Geometry: final body of the model. Coordinates: model frame, mm. A direction names the side the tool comes from. Give positions to 0.01 mm unless a question says otherwise; leave off trailing zeros. Loops run counter-clockwise (first coordinate to the right, second up) from the corner with the lowest first, then second, coordinate; pieces in that order, holes last. Notation, with made-up numbers: (5, -15) - (10, -15) arc R16 cw to (10, 3) - close; hole circle Ø1 at (-8.75, -11). An arc over 180 degrees is marked (long way). Answer in a Markdown table with one row per item.
from build123d import *
from OCP.BRepFilletAPI import BRepFilletAPI_MakeChamfer

# Parameters (mm, degrees)
SKETCH1_W            = 85
SKETCH1_H            = 23.9
BOSS_EXTRUDE1_DEPTH  = 1.7
SKETCH2_R            = 1.025
CUT_EXTRUDE1_DEPTH   = 45.180793338
SKETCH3_W            = 12
SKETCH3_H            = 6
BOSS_EXTRUDE2_DEPTH  = 5.6
SKETCH4_W            = 0.7
SKETCH4_H            = 1.5
BOSS_EXTRUDE3_DEPTH  = 3.6
CHAMFER1_SIZE        = 1.5
CHAMFER1_SIZE_2      = 1
SKETCH5_W            = 12
SKETCH5_H            = 5.6
CUT_EXTRUDE2_DEPTH   = 0.1
SKETCH6_W            = 10.2
SKETCH6_H            = 4.6
BOSS_EXTRUDE4_DEPTH  = 2.8
SKETCH7_R            = 0.7
BOSS_EXTRUDE5_DEPTH  = 5.8
BOSS_EXTRUDE6_DEPTH  = 3.65
SKETCH9_R            = 6.925
BOSS_EXTRUDE7_DEPTH  = 4.9
SKETCH10_R           = 5.95
BOSS_EXTRUDE8_DEPTH  = 4
SKETCH11_R           = 7
BOSS_EXTRUDE9_DEPTH  = 2.65
SKETCH12_R           = 4.5
CUT_EXTRUDE3_DEPTH   = 1
SKETCH13_R           = 4.45
BOSS_EXTRUDE10_DEPTH = 1.5
FILLET1_R            = 4.45
SKETCH14_W           = 13.1
SKETCH14_H           = 4.5
BOSS_EXTRUDE11_DEPTH = 2
SKETCH15_W           = 8
SKETCH15_H           = 0.5
BOSS_EXTRUDE12_DEPTH = 3


# Some blends are built 0.0001 mm under size
with BuildPart() as part:
    # Sketch1 → Boss-Extrude1 (new body)
    with BuildSketch(Plane(origin=(0, 0, 0), x_dir=(1, 0, 0), z_dir=(0, 1, 0))):
        Rectangle(SKETCH1_W, SKETCH1_H)
    extrude(amount=BOSS_EXTRUDE1_DEPTH)

    # Sketch2 → Cut-Extrude1 (cut, through all)
    with BuildSketch(Plane(origin=(0, 1.7, 0), x_dir=(1, 0, 0), z_dir=(0, 1, 0))):
        with Locations(Location((-40.605, 3.345, 0), (0, 0, 270))):
            Circle(SKETCH2_R)
        with Locations(Location((-10.45, 3.345, 0), (0, 0, 270))):
            Circle(SKETCH2_R)
        with Locations(Location((-40.605, -10.055, 0), (0, 0, 270))):
            Circle(SKETCH2_R)
        with Locations(Location((-10.45, -10.055, 0), (0, 0, 270))):
            Circle(SKETCH2_R)
        with Locations(Location((10.45, 3.345, 0), (0, 0, 270))):
            Circle(SKETCH2_R)
        with Locations(Location((40.605, 3.345, 0), (0, 0, 270))):
            Circle(SKETCH2_R)
        with Locations(Location((40.605, -10.055, 0), (0, 0, 270))):
            Circle(SKETCH2_R)
        with Locations(Location((10.45, -10.055, 0), (0, 0, 270))):
            Circle(SKETCH2_R)
    extrude(amount=-CUT_EXTRUDE1_DEPTH, mode=Mode.SUBTRACT)

    # Sketch3 → Boss-Extrude2 (add)
    with BuildSketch(Plane(origin=(0, 1.7, 0), x_dir=(1, 0, 0), z_dir=(0, 1, 0))):
        with Locations((0, 8.95)):
            Rectangle(SKETCH3_W, SKETCH3_H)
    extrude(amount=BOSS_EXTRUDE2_DEPTH)

    # Sketch4 → Boss-Extrude3 (add)
    with BuildSketch(Plane(origin=(0, 1.7, 0), x_dir=(1, 0, 0), z_dir=(0, 1, 0))):
        with Locations((-5.65, 5.2)):
            Rectangle(SKETCH4_W, SKETCH4_H)
        with Locations((5.65, 5.2)):
            Rectangle(SKETCH4_W, SKETCH4_H)
    extrude(amount=BOSS_EXTRUDE3_DEPTH)

    # Chamfer1
    chamfer1_edges_1 = [part.edges().sort_by_distance(p)[0] for p in [
        (-5.65, 5.3, -4.45),
    ]]
    chamfer1_side_1 = [part.faces().sort_by_distance(p)[0] for p in [
        (-5.65, 5.3, -4.47),
    ]]
    chamfer1_edges_2 = [part.edges().sort_by_distance(p)[0] for p in [
        (5.65, 5.3, -4.45),
    ]]
    chamfer1_side_2 = [part.faces().sort_by_distance(p)[0] for p in [
        (5.65, 5.3, -4.47),
    ]]
    chamfer1 = BRepFilletAPI_MakeChamfer(part.part.solid().wrapped)
    for e in chamfer1_edges_1:
        chamfer1.Add(CHAMFER1_SIZE - 0.0001, CHAMFER1_SIZE_2 - 0.0001, e.wrapped, chamfer1_side_1[0].wrapped)
    for e in chamfer1_edges_2:
        chamfer1.Add(CHAMFER1_SIZE - 0.0001, CHAMFER1_SIZE_2 - 0.0001, e.wrapped, chamfer1_side_2[0].wrapped)
    add(Compound.cast(chamfer1.Shape()), mode=Mode.REPLACE)  # a hair under: the kernel refuses the full size

    # Sketch5 → Cut-Extrude2 (cut)
    with BuildSketch(Plane(origin=(0, 0, -11.95), x_dir=(-1, 0, 0), z_dir=(0, 0, -1))):
        with Locations((0, 4.5)):
            Rectangle(SKETCH5_W, SKETCH5_H)
    extrude(amount=-CUT_EXTRUDE2_DEPTH, mode=Mode.SUBTRACT)

    # Sketch6 → Boss-Extrude4 (add)
    with BuildSketch(Plane(origin=(0, 0, -11.85), x_dir=(-1, 0, 0), z_dir=(0, 0, -1))):
        with Locations((0, 4.2)):
            Rectangle(SKETCH6_W, SKETCH6_H)
    extrude(amount=BOSS_EXTRUDE4_DEPTH)

    # Sketch7 → Boss-Extrude5 (add)
    with BuildSketch(Plane(origin=(0, 0, -14.65), x_dir=(-1, 0, 0), z_dir=(0, 0, -1))):
        with Locations((0.925, 4.2)):
            Circle(SKETCH7_R)
        with Locations((-0.925, 4.2)):
            Circle(SKETCH7_R)
        with Locations((-2.775, 4.2)):
            Circle(SKETCH7_R)
        with Locations((2.775, 4.2)):
            Circle(SKETCH7_R)
    extrude(amount=BOSS_EXTRUDE5_DEPTH)

    # Sketch8 → Boss-Extrude6 (add)
    with BuildSketch(Plane(origin=(0, 1.7, 0), x_dir=(1, 0, 0), z_dir=(0, 1, 0))):
        with BuildLine():
            Line((-36.5, -10.35), (-23.35, -10.35))
            Line((-23.35, -10.35), (-23.35, -5.775))
            Line((-23.35, -5.775), (-21.05, -5.775))
            ThreePointArc((-21.05, -5.775), (-19.05, -3.775), (-21.05, -1.775))
            Line((-21.05, -1.775), (-23.35, -1.775))
            Line((-23.35, -1.775), (-23.35, 2.8))
            Line((-23.35, 2.8), (-36.5, 2.8))
            Line((-36.5, 2.8), (-36.5, -1.775))
            Line((-36.5, -1.775), (-38.8, -1.775))
            ThreePointArc((-38.8, -1.775), (-40.8, -3.775), (-38.8, -5.775))
            Line((-38.8, -5.775), (-36.5, -5.775))
            Line((-36.5, -5.775), (-36.5, -10.35))
        make_face()
        with BuildLine():
            Line((23.35, -1.775), (23.35, 2.8))
            Line((23.35, 2.8), (36.5, 2.8))
            Line((36.5, 2.8), (36.5, -1.775))
            Line((36.5, -1.775), (38.8, -1.775))
            ThreePointArc((38.8, -1.775), (40.8, -3.775), (38.8, -5.775))
            Line((38.8, -5.775), (36.5, -5.775))
            Line((36.5, -5.775), (36.5, -10.35))
            Line((36.5, -10.35), (23.35, -10.35))
            Line((23.35, -10.35), (23.35, -5.775))
            Line((23.35, -5.775), (21.05, -5.775))
            ThreePointArc((21.05, -5.775), (19.05, -3.775), (21.05, -1.775))
            Line((21.05, -1.775), (23.35, -1.775))
        make_face()
    extrude(amount=BOSS_EXTRUDE6_DEPTH)

    # Sketch9 → Boss-Extrude7 (add)
    with BuildSketch(Plane(origin=(0, 5.35, 0), x_dir=(1, 0, 0), z_dir=(0, 1, 0))):
        with Locations(Location((-29.925, -3.775, 0), (0, 0, 71.706023749))):
            Circle(SKETCH9_R)
        with Locations(Location((29.925, -3.775, 0), (0, 0, 71.706023749))):
            Circle(SKETCH9_R)
    extrude(amount=BOSS_EXTRUDE7_DEPTH)

    # Sketch10 → Boss-Extrude8 (add)
    with BuildSketch(Plane(origin=(0, 10.25, 0), x_dir=(1, 0, 0), z_dir=(0, 1, 0))):
        with Locations(Location((-29.925, -3.775, 0), (0, 0, 270))):
            Circle(SKETCH10_R)
        with Locations(Location((29.925, -3.775, 0), (0, 0, 270))):
            Circle(SKETCH10_R)
    extrude(amount=BOSS_EXTRUDE8_DEPTH)

    # Sketch11 → Boss-Extrude9 (add)
    with BuildSketch(Plane(origin=(0, 14.25, 0), x_dir=(1, 0, 0), z_dir=(0, 1, 0))):
        with Locations(Location((-29.925, -3.775, 0), (0, 0, 270))):
            Circle(SKETCH11_R)
        with Locations(Location((29.925, -3.775, 0), (0, 0, 270))):
            Circle(SKETCH11_R)
    extrude(amount=BOSS_EXTRUDE9_DEPTH)

    # Sketch12 → Cut-Extrude3 (cut)
    with BuildSketch(Plane(origin=(0, 16.9, 0), x_dir=(1, 0, 0), z_dir=(0, 1, 0))):
        with Locations(Location((-29.925, -3.775, 0), (0, 0, 270))):
            Circle(SKETCH12_R)
        with Locations(Location((29.925, -3.775, 0), (0, 0, 270))):
            Circle(SKETCH12_R)
    extrude(amount=-CUT_EXTRUDE3_DEPTH, mode=Mode.SUBTRACT)

    # Sketch13 → Boss-Extrude10 (add)
    with BuildSketch(Plane(origin=(0, 15.9, 0), x_dir=(1, 0, 0), z_dir=(0, 1, 0))):
        with Locations(Location((-29.925, -3.775, 0), (0, 0, 270))):
            Circle(SKETCH13_R)
        with Locations(Location((29.925, -3.775, 0), (0, 0, 270))):
            Circle(SKETCH13_R)
    extrude(amount=BOSS_EXTRUDE10_DEPTH)

    # Fillet1
    # the kernel refuses this fillet: 4.45 mm, written as the material it takes off along each edge
    with BuildSketch(Plane(origin=(-29.925, 17.4, 3.775), x_dir=(0, 0, 1), z_dir=(-1, 0, 0))) as fillet1_piece_1:
        with BuildLine():
            CenterArc((1.11833375, -4.45), FILLET1_R, 41.52305383, 48.47694617)
            Line((1.11833375, 0), (4.45, 0))
            Line((4.45, 0), (4.45, -1.5))
        make_face()
    revolve(axis=Axis((-29.925, 17.4, 3.775), (0, 1, 0)), mode=Mode.SUBTRACT)
    with BuildSketch(Plane(origin=(29.925, 17.4, 3.775), x_dir=(0, 0, 1), z_dir=(-1, 0, 0))) as fillet1_piece_2:
        with BuildLine():
            CenterArc((1.11833375, -4.45), FILLET1_R, 41.52305383, 48.47694617)
            Line((1.11833375, 0), (4.45, 0))
            Line((4.45, 0), (4.45, -1.5))
        make_face()
    revolve(axis=Axis((29.925, 17.4, 3.775), (0, 1, 0)), mode=Mode.SUBTRACT)

    # Sketch14 → Boss-Extrude11 (add)
    with BuildSketch(Plane(origin=(0, 1.7, 0), x_dir=(1, 0, 0), z_dir=(0, 1, 0))):
        with Locations((-29.95, 9.3)):
            Rectangle(SKETCH14_W, SKETCH14_H)
        with Locations((29.95, 9.3)):
            Rectangle(SKETCH14_W, SKETCH14_H)
    extrude(amount=BOSS_EXTRUDE11_DEPTH)

    # Sketch15 → Boss-Extrude12 (add)
    with BuildSketch(Plane(origin=(0, 0, -11.55), x_dir=(-1, 0, 0), z_dir=(0, 0, -1))):
        with Locations((-29.95, 2.7)):
            Rectangle(SKETCH15_W, SKETCH15_H)
        with Locations((29.95, 2.7)):
            Rectangle(SKETCH15_W, SKETCH15_H)
    extrude(amount=BOSS_EXTRUDE12_DEPTH)


solid = part.part
Q1. Draft query along Z for faces 5 (the flat face through (23.35, 3, 8)), 6 (the cylindrical face through (-39.741, 0.862, 10.606)), 7 (the flat face through (0, 4, -5.95)). Return one class per face: pulls with the +Z half, pulls with the -Z half, needs draft (parallel to the pull), parting line crosses it, or undercut.
Check values:
| item | result |
|---|---|
| face 5 | needs draft |
| face 6 | undercut |
| face 7 | pulls with the +Z half |
Q2. First-contact query: pin 1 (2 mm diameter, centred on x = -32.5, z = -8, fed in from +Y); pin 2 (5 mm diameter, centred on x = 34.5, z = -1.5, fed in from +Y); pin 3 (2.5 mm diameter, centred on x = -37, y = 4, fed in from +Z). Flat tips, straight axial feed; report the tip coordinate or a pass-through.
Check values:
| item | result |
|---|---|
| pin 1 | y = 3.7 |
| pin 2 | y = 16.9 |
| pin 3 | z = 10.35 |
Q3. Cut plane B-B (z = -17.5). Output: boundary loops of the cut face in (x, y) (3 decimals), and give its area (3 significant figures).
Check values:
| item | result |
|---|---|
| outline | circle Ø1.4 at (-2.775, 4.2); circle Ø1.4 at (-0.925, 4.2); circle Ø1.4 at (0.925, 4.2); circle Ø1.4 at (2.775, 4.2) |
| area | 6.16 mm² |
Q4. Reachability of faces 1 (the flat face through (-30, 3, 10.35)), 2 (the flat face through (-6, 4, -8)), 3 (the flat face through (-30, 3, -2.8)), 4 (the flat face through (0, 7, -11.85)) from +Z, -Z, +X, -X, +Y, -Y: full face, straight path, thin tool, end or side. Return the list, or none.
Check values:
| item | result |
|---|---|
| face 1 | +Z, +X, -X |
| face 2 | +Z, -Z, +Y |
| face 3 | +X, -X |
| face 4 | -Z |
Q5. Cut plane A-A (x = -10.45). Output: boundary loops of the cut face in (y, z).
Check values:
| item | result |
|---|---|
| outline | (0, -11.95) - (1.7, -11.95) - (1.7, -4.37) - (0, -4.37) - close; (0, -2.32) - (1.7, -2.32) - (1.7, 9.03) - (0, 9.03) - close; (0, 11.08) - (1.7, 11.08) - (1.7, 11.95) - (0, 11.95) - close |
Q6. Material intervals for line 1 along X through (y, z) = (2, 3.5); line 2 along Z through (x, y) = (-32, 16.5); line 3 along X through (y, z) = (9, 6), sorted ascending.
Check values:
| item | result |
|---|---|
| line 1 | -40.78 to -19.07, 19.07 to 40.78 |
| line 2 | -2.91 to -0.22, 0.59 to 6.96, 7.77 to 10.46 |
| line 3 | -36.48 to -23.37, 23.37 to 36.48 |
Q7. Cut plane C-C (y = 11). Output: boundary loops of the cut face in (x, z) (3 decimals).
Check values:
| item | result |
|---|---|
| outline | circle Ø11.9 at (-29.925, 3.775); circle Ø11.9 at (29.925, 3.775) |
